Input: part model. Units: mm. Frame: model coordinates. A direction names the side the tool comes from. Round coordinates to 2 decimals unless told otherwise and drop trailing zeros. Loops run counter-clockwise (first coordinate to the right, second up) from the corner with the lowest first, then second, coordinate; pieces in that order, holes last. Notation, with made-up numbers: (-37, 83) - (-19, 83) arc R35 cw to (-19, 116) - close; hole circle Ø3 at (-2, 54). An arc over 180 degrees is marked (long way). One line per question, with ' | ' between items. Start each with the question number.
Item 1: First-contact query: pin 1 (1.5 mm diameter, centred on y = 46.5, z = 24.5, fed in from +X); pin 2 (10 mm diameter, centred on y = -45.5, z = 59.5, fed in from -X); pin 3 (10 mm diameter, centred on x = -54.5, z = 31.5, fed in from +Y); pin 4 (24 mm diameter, centred on x = 0, y = 0, fed in from +Z). Flat tips, straight axial feed; report the tip coordinate or a pass-through.
Item 2: Section A-A, the plane y = 22.5. Return loops of the section in (x, z), plus the area to 3 significant figures.
Item 3: Draft query along Z for faces 4 (the face through (40, -50, 61)), 5 (the face through (12, 14, 120)), 6 (the face through (14, -6, 35)). Return one class per face: pulls with the +Z half, pulls with the -Z half, needs draft (parallel to the pull), parting line crosses it, or undercut.
Item 4: Section C-C, the plane x = -38. Return loops of the section in (y, z), plus the area to 3 significant figures.
Item 5: Set-up query: faces 1 (the face through (-40, 50, 61)), 2 (the face through (14, -6, 85)), 3 (the face through (-40, -50, 61)). Return all of +Z, -Z, +X, -X, +Y, -Y with unobstructed straight access to the full face (end or side cutting, diameter ignored); none if empty.
Item 6: Section B-B, the plane z = 42. Return loops of the section in (x, y).
Item 7: Material intervals for line 1 along X through (y, z) = (-34, 76); line 2 along Z through (x, y) = (44.5, -2.5); line 3 along X through (y, z) = (43.5, 11), sorted ascending.
Item 8: Section D-D, the plane y = 0. Return loops of the section in (x, z), plus the area to 3 significant figures.
```python
from build123d import *

# Parameters (mm, degrees)
SKETCH1_W           = 120
SKETCH1_H           = 120
BOSS_EXTRUDE1_DEPTH = 120
SKETCH2_R           = 30
SKETCH2_W           = 20
SKETCH2_H           = 20
CUT_EXTRUDE1_DEPTH  = 120
SKETCH4_R           = 15
CUT_EXTRUDE2_DEPTH  = 120
SKETCH5_W           = 20
SKETCH5_H           = 20
CUT_EXTRUDE3_DEPTH  = 120
SKETCH6_W           = 50
SKETCH6_H           = 50
CUT_EXTRUDE4_DEPTH  = 120


with BuildPart() as part:
    # Sketch1 → Boss-Extrude1 (new body)
    with BuildSketch(Plane.XY):
        Rectangle(SKETCH1_W, SKETCH1_H)
    extrude(amount=BOSS_EXTRUDE1_DEPTH)

    # Sketch2 → Cut-Extrude1 (cut)
    with BuildSketch(Plane.XY.offset(120)):
        with Locations((0, -60)):
            Circle(SKETCH2_R)
        with Locations((50, -50)):
            Rectangle(SKETCH2_W, SKETCH2_H)
        with Locations((-50, -50)):
            Rectangle(SKETCH2_W, SKETCH2_H)
    extrude(amount=-CUT_EXTRUDE1_DEPTH, mode=Mode.SUBTRACT)

    # Sketch4 → Cut-Extrude2 (cut)
    with BuildSketch(Plane.XY.offset(120)):
        Circle(SKETCH4_R)
    extrude(amount=-CUT_EXTRUDE2_DEPTH, mode=Mode.SUBTRACT)

    # Sketch5 → Cut-Extrude3 (cut)
    with BuildSketch(Plane.XY.offset(120)):
        with Locations((-50, 50)):
            Rectangle(SKETCH5_W, SKETCH5_H)
        with BuildLine():
            Line((0, 60), (-12.5, 60))
            ThreePointArc((-12.5, 60), (-8.838834765, 51.161165235), (0, 47.5))
            Line((0, 47.5), (0, 60))
        make_face()
        with BuildLine():
            Line((0, 60), (0, 47.5))
            ThreePointArc((0, 47.5), (8.838834765, 51.161165235), (12.5, 60))
            Line((12.5, 60), (0, 60))
        make_face()
        with Locations((50, 50)):
            Rectangle(SKETCH5_W, SKETCH5_H)
    extrude(amount=-CUT_EXTRUDE3_DEPTH, mode=Mode.SUBTRACT)

    # Sketch6 → Cut-Extrude4 (cut)
    with BuildSketch(Plane(origin=(60, 0, 0), x_dir=(0, 0, -1), z_dir=(1, 0, 0))):
        with Locations((-60, 0)):
            Rectangle(SKETCH6_W, SKETCH6_H)
    extrude(amount=-CUT_EXTRUDE4_DEPTH, mode=Mode.SUBTRACT)


solid = part.part
```
Return value:
1) pin 1: x = 40 | pin 2: x = -40 | pin 3: y = 40 | pin 4: through
2) outline: (-60, 0) - (60, 0) - (60, 35) - (-60, 35) - close; (-60, 85) - (60, 85) - (60, 120) - (-60, 120) - close | area: 8,400 mm2
3) face 4: needs draft | face 5: pulls with the +Z half | face 6: undercut
4) outline: (-60, 0) - (60, 0) - (60, 120) - (-60, 120) - close; hole (-25, 35) - (25, 35) - (25, 85) - (-25, 85) - close | area: 11,900 mm2
5) face 1: +Z, -Z, -X, +Y | face 2: +X, -X | face 3: +Z, -Z, -X, -Y
6) outline: (-60, -40) - (-40, -40) - (-40, -60) - (-30, -60) arc R30 cw to (30, -60) - (40, -60) - (40, -40) - (60, -40) - (60, -25) - (-60, -25) - close; (-60, 25) - (60, 25) - (60, 40) - (40, 40) - (40, 60) - (12.5, 60) arc R12.5 cw to (-12.5, 60) - (-40, 60) - (-40, 40) - (-60, 40) - close
7) line 1: -60 to -14.97, 14.97 to 60 | line 2: 0 to 35, 85 to 120 | line 3: -40 to 40
8) outline: (-60, 0) - (-15, 0) - (-15, 35) - (-60, 35) - close; (-60, 85) - (-15, 85) - (-15, 120) - (-60, 120) - close; (15, 0) - (60, 0) - (60, 35) - (15, 35) - close; (15, 85) - (60, 85) - (60, 120) - (15, 120) - close | area: 6,300 mm2
